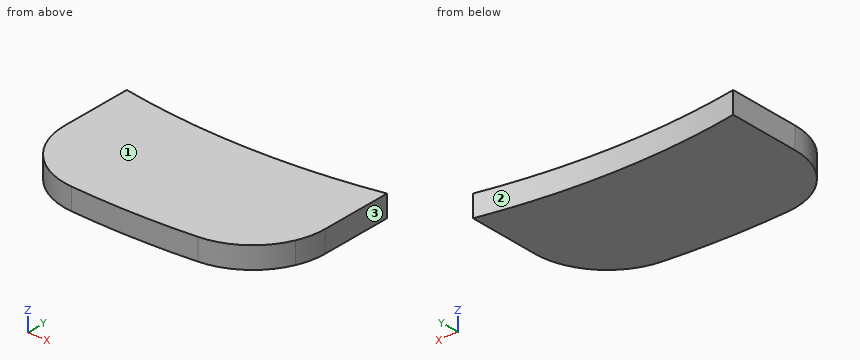
```python
from build123d import *

# Parameters (mm, degrees)
BOSS_EXTRUDE1_DEPTH = 3


with BuildPart() as part:
    # Sketch2 → Boss-Extrude1 (new body)
    with BuildSketch(Plane.XY):
        with BuildLine():
            Line((18, -104.694794522), (18, -94.399205505))
            ThreePointArc((18, -94.399205505), (0, -96.1), (-18, -94.399205505))
            Line((-18, -94.399205505), (-18, -104.694794522))
            ThreePointArc((-18, -104.694794522), (-15.335497516, -111.49115209), (-8.761904762, -114.665727334))
            ThreePointArc((-8.761904762, -114.665727334), (0, -115), (8.761904762, -114.665727334))
            ThreePointArc((8.761904762, -114.665727334), (13.812374448, -112.832134584), (17.184851944, -108.649348197))
            ThreePointArc((17.184851944, -108.649348197), (17.794093103, -106.713640797), (18, -104.694794522))
        make_face()
    extrude(amount=BOSS_EXTRUDE1_DEPTH)


solid = part.part
```
Build history of the part. All positions in model axes, mm. Face numbers are marked on the shaded views. Round coordinates to 2 decimals unless told otherwise and drop trailing zeros. Write each loop counter-clockwise with the first axis right and the second up, starting at its lowest first coordinate (ties: lowest second). Pieces come first, ordered by that corner, then holes.
1) Band-saw the part on C-C, the plane y = -107.5. List the corners of the cut face in (x, z).
2) Band-saw the part on A-A, the plane z = 1. List the corners of the cut face in (x, y), and give its area (3 significant figures).
3) Drill centre lines: probe 1 along Y at (x, z) = (8.5, 1.05); probe 2 along Y at (x, z) = (-14, 1.9); probe 3 along X at (y, z) = (-108, 1.1). Where is each one in solid material? Low to high.
4) Pin check, flat tips, straight feed: pin 1 (1.5 mm diameter, centred on y = -109, z = 2, fed in from +X); pin 2 (1.5 mm diameter, centred on y = -110.5, z = 2, fed in from +X); pin 3 (1 mm diameter, centred on x = 10, z = 1.5, fed in from -Y). Stop position of each tip, or through.
5) Band-saw the part on B-B, the plane x = 0. List the corners of the cut face in (y, z), and give its area (3 significant figures).
6) Mould opens along X. For the marked faces 1, 2 and 3 say: +X half, -X half, draft (parallel to the pull), parting line (faces both ways), or undercut.
Ans:
1. outline: (-17.6, 0) - (17.6, 0) - (17.6, 3) - (-17.6, 3) - close
2. outline: (-18, -104.69) arc R10 ccw to (-8.76, -114.67) arc R115 ccw to (8.76, -114.67) arc R10 ccw to (18, -104.69) - (18, -94.4) arc R96.1 cw to (-18, -94.4) - close
2. area: 650 mm2
3. probe 1: y = -114.69 to -95.72
3. probe 2: y = -112.69 to -95.07
3. probe 3: x = -17.44 to 17.44
4. pin 1: stops at x = 17.35
4. pin 2: stops at x = 16.63
4. pin 3: stops at y = -114.58
5. outline: (-115, 0) - (-96.1, 0) - (-96.1, 3) - (-115, 3) - close
5. area: 56.7 mm2
6. face 1: draft
6. face 2: undercut
6. face 3: +X half
